```python
from build123d import *

# Parameters (mm, degrees)
F0_W      = 58.42
F0_H      = 45.72
F1_DEPTH  = 3.81
F2_W      = 58.42
F2_H      = 5.08
F3_DEPTH  = 38.1
F4_R      = 1.905
F5_DEPTH  = 3.811
F6_W      = 10.16
F6_H      = 10.16
F7_DEPTH  = 5.08
F8_SIZE   = 10.15999
F9_W      = 10.16
F9_H      = 10.16
F10_DEPTH = 5.08
F11_SIZE  = 10.15999


# Not quite as in the source:
# - a fillet or chamfer is up to 0.001 mm smaller than in the source, because OpenCascade refuses the exact size


with BuildPart() as f1:
    # F0 (on Top) → F1 (new body)
    with BuildSketch(Plane.XY):
        Rectangle(F0_W, F0_H)
    extrude(amount=F1_DEPTH)

    # F2 (on face) → F3 (join)
    with BuildSketch(Plane.XY.offset(3.81)):
        with Locations((0, -20.32)):
            Rectangle(F2_W, F2_H)
    extrude(amount=F3_DEPTH)

    # F4 (on face) → F5 (cut, through all)
    with BuildSketch(Plane.XY.offset(3.81)):
        with Locations((-14.224, 17.78)):
            Circle(F4_R)
        with Locations((14.224, 17.78)):
            Circle(F4_R)
        with Locations((14.224, -10.668)):
            Circle(F4_R)
        with Locations((-14.224, -10.668)):
            Circle(F4_R)
    extrude(amount=-F5_DEPTH, mode=Mode.SUBTRACT)

    # F6 (on face) → F7 (join)
    with BuildSketch(Plane(origin=(-29.21, 0, 0), x_dir=(0, -1, 0), z_dir=(-1, 0, 0))):
        with Locations((12.7, 8.89)):
            Rectangle(F6_W, F6_H)
    extrude(amount=-F7_DEPTH)

    # F8 (size 10.16 in the source; OpenCascade refuses exactly that, so slightly less here)
    f8_edges = [f1.edges().sort_by_distance(p)[0] for p in [
        (-26.67, -7.62, 13.97),
    ]]
    chamfer(f8_edges, length=F8_SIZE)

    # F9 (on face) → F10 (join)
    with BuildSketch(Plane.YZ.offset(29.21)):
        with Locations((-12.7, 8.89)):
            Rectangle(F9_W, F9_H)
    extrude(amount=-F10_DEPTH)

    # F11 (size 10.16 in the source; OpenCascade refuses exactly that, so slightly less here)
    f11_edges = [f1.edges().sort_by_distance(p)[0] for p in [
        (26.67, -7.62, 13.97),
    ]]
    chamfer(f11_edges, length=F11_SIZE)


solid = f1.part
```
Geometry check sheet. Reference: the model listing, model coordinates, mm. A direction names the side the tool comes from. Coordinates: 2 decimals unless noted, no trailing zeros. Order: outer loops, then holes, each group sorted by start corner. A loop starts at its lowest first (then second) coordinate and runs counter-clockwise, first axis right, second up. Notation, with made-up numbers: (-4, 87) - (9, 87) arc R32 cw to (9, 121) - close; hole circle Ø3 at (3, -3). An arc over 180 degrees is marked (long way). Answer in a Markdown table with one row per item. Add a question column.
1. Section check C-C (x = -15). Enter the section's corners in (y, z).
2. Material ranges on L1, parallel to X at y = 17, z = 2; L2, parallel to Z at x = 23.5, y = 6; L3, parallel to Y at x = -7, z = 25.5, recorded low to high. Write a range as [from, to].
3. Section check B-B (x = 10). Enter the section's corners in (y, z), plus the area to 3 significant figures.
4. Draft check along Y on faces 3 (the face through (-13.2, -9.06, 1.93)), 4 (the face through (0, -17.78, 23)), 5 (the face through (-24.13, -15, 7)), 6 (the face through (0, -22.86, 21)). Enter one of: +Y half, -Y half, draft (parallel to the pull), parting line (faces both ways), or undercut.
5. Access from +Z, -Z, +X, -X, +Y, -Y to the whole of each face (thin tool, end or side, straight path). Record for faces 1 (the face through (0, 3, 3.81)), 2 (the face through (-26.71, -12.77, 8.96)).
6. Section check A-A (y = 17.78). Enter the section's corners in (x, z).
7. Section check D-D (z = 13). Enter the section's corners in (x, y), plus the area to 3 significant figures.
8. Gauge pin test, flat ends, axial feed: pin 1 Ø6 at (x, y) = (-14.224, -10.668) entering from -Z; pin 2 Ø8 at (x, z) = (1, 25) entering from +Y; pin 3 Ø3 at (x, y) = (14.224, -10.668) entering from -Z; pin 4 Ø12 at (x, y) = (7, -7) entering from +Z. Record the tip position at first contact, or that the pin passes through.
Data:
| question | item | result |
|---|---|---|
| 1 | outline | (-22.86, 0) - (-12.41, 0) - (-12.41, 3.81) - (-17.78, 3.81) - (-17.78, 41.91) - (-22.86, 41.91) - close; (-8.93, 0) - (16.04, 0) - (16.04, 3.81) - (-8.93, 3.81) - close; (19.52, 0) - (22.86, 0) - (22.86, 3.81) - (19.52, 3.81) - close |
| 2 | L1 | x = [-29.21, -15.96], [-12.49, 12.49], [15.96, 29.21] |
| 2 | L2 | z = [0, 3.81] |
| 2 | L3 | y = [-22.86, -17.78] |
| 3 | outline | (-22.86, 0) - (22.86, 0) - (22.86, 3.81) - (-17.78, 3.81) - (-17.78, 41.91) - (-22.86, 41.91) - close |
| 3 | area | 368 mm² |
| 4 | face 3 | undercut |
| 4 | face 4 | +Y half |
| 4 | face 5 | draft |
| 4 | face 6 | -Y half |
| 5 | face 1 | +Z, +Y |
| 5 | face 2 | +Z, +X, -X, +Y |
| 6 | outline | (-29.21, 0) - (-16.13, 0) - (-16.13, 3.81) - (-29.21, 3.81) - close; (-12.32, 0) - (12.32, 0) - (12.32, 3.81) - (-12.32, 3.81) - close; (16.13, 0) - (29.21, 0) - (29.21, 3.81) - (16.13, 3.81) - close |
| 7 | outline | (-29.21, -22.86) - (29.21, -22.86) - (29.21, -16.81) - (24.13, -16.81) - (24.13, -17.78) - (-24.13, -17.78) - (-24.13, -16.81) - (-29.21, -16.81) - close |
| 7 | area | 307 mm² |
| 8 | pin 1 | stops at z = 0 |
| 8 | pin 2 | stops at y = -17.78 |
| 8 | pin 3 | passes through |
| 8 | pin 4 | stops at z = 3.81 |
